The model under review builds one solid part; all positions refer to its coordinate system, in mm. A direction names the side the tool comes from. Give positions to 0.01 mm unless a question says otherwise; leave off trailing zeros. Loops run counter-clockwise (first coordinate to the right, second up) from the corner with the lowest first, then second, coordinate; pieces in that order, holes last. Notation, with made-up numbers: M 16.5,25 L 49.5,25 A19 ccw 49.5,61 Z; hole C -12,84 d1. An arc over 180 degrees is marked long. One line per item, written item: value. Start each with the question number.
Q1. We need section B-B on z = 2.9. Give the number of separate pieces and of enclosed holes in the cut face, plus the area to 3 significant figures.
Q2. We need section D-D on y = 20. Write out the cut boundary in (x, z), plus the area to 3 significant figures.
Q3. We need section C-C on x = -45. Write out the cut boundary in (y, z).
Q4. To check wall thickness, follow line 1 along Y through (x, z) = (45, 1.55); line 2 along X through (y, z) = (-3, 1.3); line 3 along X through (y, z) = (19, 1.2). State the ranges of each line that lie inside material, in increasing order. Write a range as from..to.
Q5. For faces 1 (the face through (-50, 42, 2)), 2 (the face through (-36.83, -7, 2)), list the 3-axis set-ups (+Z, -Z, +X, -X, +Y, -Y) from which the entire face can be reached by the end or side of a thin tool; tool diameter is ignored.
Q6. Mouldability with a two-part tool opening along Y and no side actions: class faces 3 (the face through (-1, 100, 2)), 4 (the face through (47.31, 59.04, 2.46)), 5 (the face through (47.31, 79.04, 2.46)), 6 (the face through (1, 56, 0)) as released by +Y, released by -Y, zero draft, split by the parting line, or undercut.
Q7. For pin 1 (1.5 mm diameter, centred on x = -9, z = 2, fed in from -Y), flat-tipped, find the tip position at first contact; note if it passes through.
Q8. We need section A-A on y = 40. Write out the cut boundary in (x, z), plus the area to 3 significant figures.
```python
from build123d import *

# Parameters (mm, degrees)
SKETCH1_R           = 2.5
BOSS_EXTRUDE1_DEPTH = 5


with BuildPart() as part:
    # Sketch1 → Boss-Extrude1 (new body)
    with BuildSketch(Plane.XY):
        with BuildLine():
            Line((-50, -15), (-50, 100))
            Line((-50, 100), (50, 100))
            Line((50, 100), (50, -15))
            Line((50, -15), (36.83, -15))
            Line((36.83, -15), (36.83, 0))
            ThreePointArc((36.83, 0), (0, 36.83), (-36.83, 0))
            Line((-36.83, 0), (-36.83, -15))
            Line((-36.83, -15), (-50, -15))
        make_face()
        with Locations((-45, 0)):
            Circle(SKETCH1_R, mode=Mode.SUBTRACT)
        with Locations((45, 0)):
            Circle(SKETCH1_R, mode=Mode.SUBTRACT)
        with Locations((45, 20)):
            Circle(SKETCH1_R, mode=Mode.SUBTRACT)
        with Locations((45, 40)):
            Circle(SKETCH1_R, mode=Mode.SUBTRACT)
        with Locations((45, 60)):
            Circle(SKETCH1_R, mode=Mode.SUBTRACT)
        with Locations((45, 80)):
            Circle(SKETCH1_R, mode=Mode.SUBTRACT)
        with Locations((-45, 20)):
            Circle(SKETCH1_R, mode=Mode.SUBTRACT)
        with Locations((-45, 40)):
            Circle(SKETCH1_R, mode=Mode.SUBTRACT)
        with Locations((-45, 60)):
            Circle(SKETCH1_R, mode=Mode.SUBTRACT)
        with Locations((-45, 80)):
            Circle(SKETCH1_R, mode=Mode.SUBTRACT)
    extrude(amount=BOSS_EXTRUDE1_DEPTH)


solid = part.part
```
Solved:
1. separate pieces: 1
1. enclosed holes: 10
1. area: 8,070 mm2
2. outline: M -50,0 L -47.5,0 L -47.5,5 L -50,5 Z; M -42.5,0 L -30.93,0 L -30.93,5 L -42.5,5 Z; M 30.93,0 L 42.5,0 L 42.5,5 L 30.93,5 Z; M 47.5,0 L 50,0 L 50,5 L 47.5,5 Z
2. area: 141 mm2
3. outline: M -15,0 L -2.5,0 L -2.5,5 L -15,5 Z; M 2.5,0 L 17.5,0 L 17.5,5 L 2.5,5 Z; M 22.5,0 L 37.5,0 L 37.5,5 L 22.5,5 Z; M 42.5,0 L 57.5,0 L 57.5,5 L 42.5,5 Z; M 62.5,0 L 77.5,0 L 77.5,5 L 62.5,5 Z; M 82.5,0 L 100,0 L 100,5 L 82.5,5 Z
4. line 1: -15..-2.5, 2.5..17.5, 22.5..37.5, 42.5..57.5, 62.5..77.5, 82.5..100
4. line 2: -50..-36.83, 36.83..50
4. line 3: -50..-47.29, -42.71..-31.55, 31.55..42.71, 47.29..50
5. face 1: +Z, -Z, -X, +Y, -Y
5. face 2: +Z, -Z, -Y
6. face 3: released by +Y
6. face 4: undercut
6. face 5: undercut
6. face 6: zero draft
7. pin 1: y = 35.52
8. outline: M -50,0 L -47.5,0 L -47.5,5 L -50,5 Z; M -42.5,0 L 42.5,0 L 42.5,5 L -42.5,5 Z; M 47.5,0 L 50,0 L 50,5 L 47.5,5 Z
8. area: 450 mm2
